Part print with two shaded views. Sizes in mm from the minimum x, y, z corner. A direction names the side the tool comes from. Give positions to 0.01 mm unless a question says otherwise; leave off trailing zeros. Order: outer loops, then holes, each group sorted by start corner. A loop starts at its lowest first (then second) coordinate and runs counter-clockwise, first axis right, second up. Notation, with made-up numbers: (-0.5, -33.5) - (29.5, -33.5) arc R13 ccw to (29.5, -8.5) - close; hole circle Ø4 at (77.25, 88). An arc over 180 degrees is marked (long way). Return JSON: item names as keys, results as strings. Group by question number.
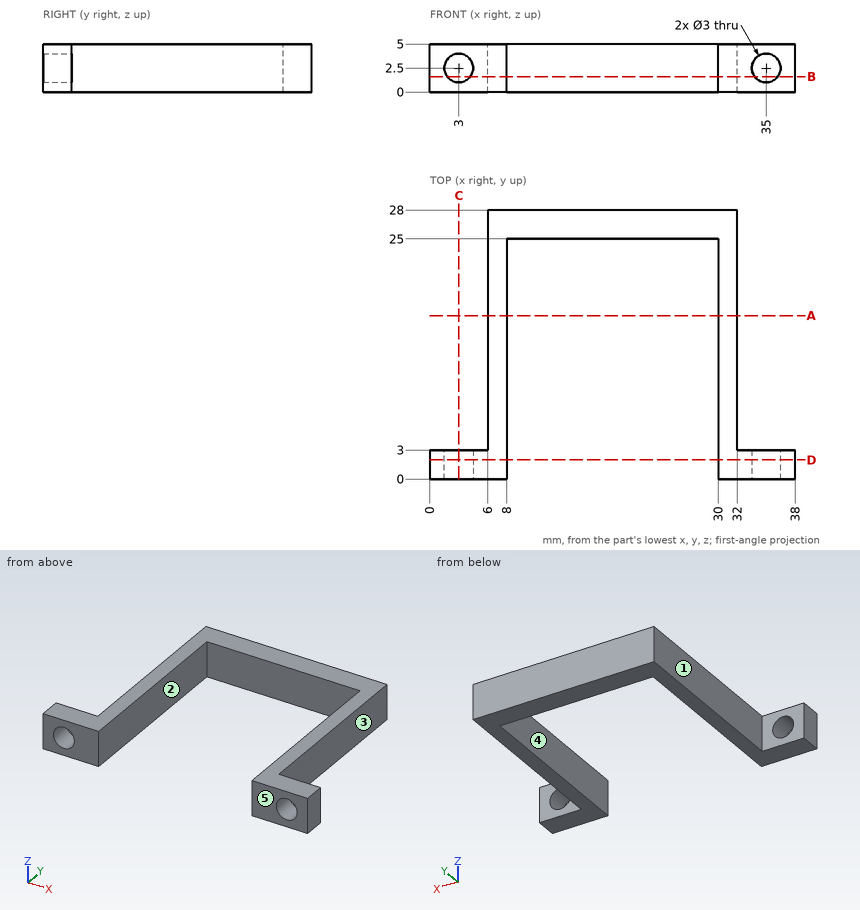
(1) Slice it at C-C (x = 3). Give the cut face in (y, z), and give its area (3 significant figures).
(2) Drop flat-ended pins along their axis: pin 1 Ø1.5 at (x, z) = (2, 3) entering from +Y; pin 2 Ø2 at (y, z) = (12.5, 2) entering from +X; pin 3 Ø2.5 at (y, z) = (16.5, 2.5) entering from -X. Give the stop position or say it passes through.
(3) Slice it at D-D (y = 2). Give the cut face in (x, z), and give its area (3 significant figures).
(4) Drill centre lines: L1, parallel to X at y = 1.3, z = 2.5; L2, parallel to Z at x = 3, y = 1.15; L3, parallel to X at y = 17.5, z = 2.5. Where is each one in solid material? Low to high.
(5) Slice it at A-A (y = 17). Give the cut face in (x, z), and give its area (3 significant figures).
(6) 3-axis set-ups, long thin cutter, end or side, ignore diameter. For the marked faces 4 and 5: which of +Z, -Z, +X, -X, +Y, -Y reach the whole face in a straight line?
(7) Slice it at B-B (z = 1.6). Give the cut face in (x, y).
(8) Pull direction X, two halves, no side cores. Call the marked faces 1, 2 and 3: released by +X, released by -X, zero draft, split by the parting line, or undercut.
Result set:
{
 "1": {"outline": "(0, 0) - (3, 0) - (3, 1) - (0, 1) - close; (0, 4) - (3, 4) - (3, 5) - (0, 5) - close", "area": "6.00 mm²"},
 "2": {"pin 1": "stops at y = 3", "pin 2": "stops at x = 32", "pin 3": "stops at x = 6"},
 "3": {"outline": "(0, 0) - (8, 0) - (8, 5) - (0, 5) - close; (30, 0) - (38, 0) - (38, 5) - (30, 5) - close; hole circle Ø3 at (3, 2.5); hole circle Ø3 at (35, 2.5)", "area": "65.9 mm²"},
 "4": {"L1": "x = 0 to 1.5, 4.5 to 8, 30 to 33.5, 36.5 to 38", "L2": "z = 0 to 1, 4 to 5", "L3": "x = 6 to 8, 30 to 32"},
 "5": {"outline": "(6, 0) - (8, 0) - (8, 5) - (6, 5) - close; (30, 0) - (32, 0) - (32, 5) - (30, 5) - close", "area": "20.0 mm²"},
 "6": {"face 4": "+Z, -Z, -Y", "face 5": "+Z, -Z, +X, -X, -Y"},
 "7": {"outline": "(0, 0) - (1.8, 0) - (1.8, 3) - (0, 3) - close; (4.2, 0) - (8, 0) - (8, 25) - (30, 25) - (30, 0) - (33.8, 0) - (33.8, 3) - (32, 3) - (32, 28) - (6, 28) - (6, 3) - (4.2, 3) - close; (36.2, 0) - (38, 0) - (38, 3) - (36.2, 3) - close"},
 "8": {"face 1": "released by -X", "face 2": "undercut", "face 3": "released by +X"}
}
